```python
from build123d import *

# Parameters (mm, degrees)
ESQUISSE1_R                  = 13
BASE_EXTRUSION_DEPTH         = 1
BOSS_EXTRU_MINCE1_DEPTH      = 2
R_P_TITION_CIRCULAIRE1_COUNT = 10
R_P_TITION_CIRCULAIRE1_ANGLE = 294.545454545
BOSS_EXTRU_MINCE2_DEPTH      = 2


with BuildPart() as part:
    # Esquisse1 → Base-Extrusion (new body)
    with BuildSketch(Plane.XY):
        Circle(ESQUISSE1_R)
        with BuildLine():
            Line((-2, 8.5), (2, 8.5))
            Line((2, 8.5), (2, 9.797958971))
            ThreePointArc((2, 9.797958971), (0, -10), (-2, 9.797958971))
            Line((-2, 9.797958971), (-2, 8.5))
        make_face(mode=Mode.SUBTRACT)
    extrude(amount=BASE_EXTRUSION_DEPTH)

    # Esquisse2 → Boss.-Extru.-Mince1 (add, symmetric)
    with BuildSketch(Plane(origin=(0, 0, 0), x_dir=(-0.5406408174555986, 0.8412535328311805, 0), z_dir=(0.8412535328311805, 0.5406408174555986, 0))):
        with BuildLine():
            Line((10, 0), (13, 0))
            ThreePointArc((13, 0), (13.216439614, 0.023703993), (13.422618262, 0.093692213))
            Line((13.422618262, 0.093692213), (18, 2.228160372))
            Line((18, 2.228160372), (17.577381738, 3.134468159))
            Line((17.577381738, 3.134468159), (13, 1))
            Line((13, 1), (10, 1))
            Line((10, 1), (10, 0))
        make_face()
    boss_extru_mince1 = extrude(amount=BOSS_EXTRU_MINCE1_DEPTH, both=True)

    # Répétition circulaire1: Boss.-Extru.-Mince1 ×10 about axis
    r_p_tition_circulaire1_axis = Axis((0, 0, -7.805907173), (0, 0, 1))
    for i in range(1, R_P_TITION_CIRCULAIRE1_COUNT):
        add(boss_extru_mince1.rotate(r_p_tition_circulaire1_axis, i * R_P_TITION_CIRCULAIRE1_ANGLE / (R_P_TITION_CIRCULAIRE1_COUNT - 1)))

    # Esquisse3 → Boss.-Extru.-Mince2 (add, symmetric)
    with BuildSketch(Plane(origin=(0, 0, 0), x_dir=(0, 0, -1), z_dir=(1, 0, 0))):
        with BuildLine():
            Line((0, 10), (0, 13))
            ThreePointArc((0, 13), (-0.034074174, 13.258819045), (-0.133974596, 13.5))
            Line((-0.133974596, 13.5), (-0.711324865, 14.5))
            ThreePointArc((-0.711324865, 14.5), (-1.077350269, 14.866025404), (-1.577350269, 15))
            Line((-1.577350269, 15), (-5.577350269, 15))
            Line((-5.577350269, 15), (-5.577350269, 14))
            Line((-5.577350269, 14), (-1.577350269, 14))
            Line((-1.577350269, 14), (-1, 13))
            Line((-1, 13), (-1, 10))
            Line((-1, 10), (0, 10))
        make_face()
    extrude(amount=BOSS_EXTRU_MINCE2_DEPTH, both=True)


solid = part.part
```
Check sheet for the modelled part. Datum: model origin and axes. Units: mm. A direction names the side the tool comes from. Round coordinates to 2 decimals unless told otherwise and drop trailing zeros. Write each loop counter-clockwise with the first axis right and the second up, starting at its lowest first coordinate (ties: lowest second). Pieces come first, ordered by that corner, then holes. Notation, with made-up numbers: M 19.25,25 L 45.25,25 A32 cw 45.25,58 Z; hole C -5.75,73.5 d8. An arc over 180 degrees is marked long. Write item = value, one per line. Start each with the question number.
1. Section check B-B, the plane x = 9.5. State how many separate pieces and enclosed holes the cut face has, then the cut area to 3 significant figures.
2. Gauge pin test, flat ends, axial feed: pin 1 (0.6 mm diameter, centred on y = 14, z = 2.5, fed in from +X); pin 2 (2 mm diameter, centred on x = 1, z = 3.5, fed in from +Y); pin 3 (16 mm diameter, centred on x = 0, y = 0, fed in from +Z); pin 4 (1.1 mm diameter, centred on y = 9.5, z = 0.5, fed in from +X). Record the tip position at first contact, or that the pin passes through.
3. Tool access check on faces 4 (the flat face through (-11.597, -10.012, 2.082)), 5 (the cylindrical face through (9.84, 8.495, 0.493)), 6 (the flat face through (10.01, 11.88, 1.57)). Record the directions out of +Z, -Z, +X, -X, +Y, -Y that give a thin tool (end or side, any length) a straight path to the whole face; none if there is none.
4. Release check for a two-part mould opening along X. For faces 1 (the flat face through (-14.969, -4.173, 1.575)), 2 (the flat face through (11.831, -10.289, 1.146)), 3 (the flat face through (-6.26, -14.22, 1.57)) record: pulls with the +X half, pulls with the -X half, needs draft (parallel to the pull), parting line crosses it, or undercut.
5. Section check A-A, the plane x = 0. Record the cut outline in (y, z).
6. Scan lines: line 1 (Y direction, x = 0, z = 3.35); line 2 (Y direction, x = 0, z = 0.65); line 3 (Y direction, x = 0, z = 0.55). Record each from-to range of solid material in increasing order. Write a range as [from, to].
Results found:
q1.separate_pieces = 3
q1.enclosed_holes = 0
q1.area = 18.1 mm^2
q2.pin_1 = 11.41
q2.pin_2 = 15
q2.pin_3 = through
q2.pin_4 = 9.43
q3.face_4 = +Z
q3.face_5 = +Z, -Z
q3.face_6 = +Z, -Z, +X
q4.face_1 = undercut
q4.face_2 = pulls with the +X half
q4.face_3 = pulls with the -X half
q5.outline = M -13,0 L -10,0 L -10,1 L -13,1 Z; M 8.5,0 L 13,0 A1 ccw 13.5,0.13 L 14.5,0.71 A1 ccw 15,1.58 L 15,5.58 L 14,5.58 L 14,1.58 L 13,1 L 8.5,1 Z
q6.line_1 = [14, 15]
q6.line_2 = [-13, -10], [8.5, 14.39]
q6.line_3 = [-13, -10], [8.5, 14.22]
